Source: CAD feature listing. Evaluate the final solid. Frame: model axes, mm. A direction names the side the tool comes from. Round coordinates to 2 decimals unless told otherwise and drop trailing zeros. Order: outer loops, then holes, each group sorted by start corner. A loop starts at its lowest first (then second) coordinate and runs counter-clockwise, first axis right, second up. Notation, with made-up numbers: (8, 8) - (44, 8) arc R9 cw to (44, 12) - close; hole circle Ø10 at (27.5, 3). An arc over 180 degrees is marked (long way). Return JSON: item names as keys, results as strings. Group by question number.
1) Access query for faces 1 (the flat face through (150, -44, 49)), 2 (the flat face through (154, 38, 66)), 3 (the flat face through (140, -41, 59)). Directions: +Z, -Z, +X, -X, +Y, -Y. A direction counts if a zero-diameter tool reaches every point of the face in a straight line with its end or side. Return the directions, or none.
2) Section A-A, the plane x = 139.5. Return loops of the section in (y, z), plus the area to 3 significant figures.
3) Section D-D, the plane x = 164.5. Return loops of the section in (y, z).
4) Ray query, line 1 (Y direction, x = 139.5, z = 56); line 2 (Y direction, x = 153, z = 52.5); line 3 (Z direction, x = 159, y = -23). Return the intervals inside material, ascending. Write a range as from..to.
5) Mould query, pull axis Y, two halves, no side actions, for faces 4 (the flat face through (154, -50, 72)), 5 (the flat face through (150, 44, 49)), 6 (the cylindrical face through (137.199, -46.265, 54.07)). Classes: pulls with the +Y half, pulls with the -Y half, needs draft (parallel to the pull), parting line crosses it, or undercut.
6) Section C-C, the plane y = 43. Return loops of the section in (x, z).
7) Contact query for flat-ended pins moving along their axis: P1, Ø2, axis at y = -39.5, z = 69.5, coming from the -X side; P2, Ø6.5, axis at x = 139.5, y = -44.5, coming from the +Z side; P3, Ø3, axis at y = 35.5, z = 89.5, coming from the -X side (3 decimals); P4, Ø5, axis at x = 148.5, y = 28.5, coming from the -Z side. Output: stop coordinate, or through.
8) Section B-B, the plane z = 63.5. Return loops of the section in (x, y).
```python
from build123d import *

# Parameters (mm, degrees)
SKETCH132_W   = 12
SKETCH132_H   = 44
SKETCH132_W_2 = 100
SKETCH132_H_2 = 16
PAD051_DEPTH  = 20
SKETCH134_W   = 15
SKETCH134_H   = 12
PAD052_DEPTH  = 10
SKETCH133_R   = 2.9
HOLE008_DEPTH = 25


with BuildPart() as part:
    # Sketch132 → Pad051 (new body)
    with BuildSketch(Plane.YZ):
        with Locations((-42, 60)):
            Rectangle(SKETCH132_W, SKETCH132_H)
        with Locations((46, 60)):
            Rectangle(SKETCH132_W, SKETCH132_H)
        with Locations((2, 90)):
            Rectangle(SKETCH132_W_2, SKETCH132_H_2)
    extrude(amount=PAD051_DEPTH)

    # Sketch134 → Pad052 (join)
    with BuildSketch(Plane.XY.offset(38)):
        with Locations((-6.5, -42)):
            Rectangle(SKETCH134_W, SKETCH134_H)
        with Locations((-6.5, 46)):
            Rectangle(SKETCH134_W, SKETCH134_H)
    extrude(amount=PAD052_DEPTH)

    # Sketch133 → Hole008 (cut)
    with BuildSketch(Plane.XY.offset(48)):
        with Locations((-7.5, 45)):
            Circle(SKETCH133_R)
        with Locations((-7.5, -42.5)):
            Circle(SKETCH133_R)
    extrude(amount=-HOLE008_DEPTH, mode=Mode.SUBTRACT)


with BuildPart() as part_1:
    # Body080 placement: moved
    add(part.part.moved(Location((147, -2, 11))))


solid = part_1.part
```
Geometry check:
{
 "1": {"face 1": "-Z, +X, -X, +Y, -Y", "face 2": "-Z, +X, -X", "face 3": "+Z, -X, +Y, -Y"},
 "2": {"outline": "(-50, 49) - (-47.4, 49) - (-47.4, 59) - (-50, 59) - close; (-41.6, 49) - (-38, 49) - (-38, 59) - (-41.6, 59) - close; (38, 49) - (40.1, 49) - (40.1, 59) - (38, 59) - close; (45.9, 49) - (50, 49) - (50, 59) - (45.9, 59) - close", "area": "124 mm2"},
 "3": {"outline": "(-50, 49) - (-38, 49) - (-38, 93) - (38, 93) - (38, 49) - (50, 49) - (50, 109) - (-50, 109) - close"},
 "4": {"line 1": "-50..-47.4, -41.6..-38, 38..40.1, 45.9..50", "line 2": "-50..-38, 38..50", "line 3": "93..109"},
 "5": {"face 4": "pulls with the -Y half", "face 5": "needs draft", "face 6": "undercut"},
 "6": {"outline": "(133, 49) - (136.6, 49) - (136.6, 59) - (133, 59) - close; (142.4, 49) - (167, 49) - (167, 109) - (147, 109) - (147, 59) - (142.4, 59) - close"},
 "7": {"P1": "x = 147", "P2": "z = 59", "P3": "through", "P4": "z = 93"},
 "8": {"outline": "(147, -50) - (167, -50) - (167, -38) - (147, -38) - close; (147, 38) - (167, 38) - (167, 50) - (147, 50) - close"}
}
